Print and shaded views of the part. All mm, measured from the part's lowest x, y and z. Give positions to 0.01 mm unless a question says otherwise; leave off trailing zeros. Loops run counter-clockwise (first coordinate to the right, second up) from the corner with the lowest first, then second, coordinate; pieces in that order, holes last. Notation, with made-up numbers: (-7, -1.75) - (35, -1.75) arc R23 ccw to (35, 11.25) - close; hole circle Ø9 at (72, 4). An arc over 180 degrees is marked (long way). Return JSON: item names as keys, results as strings.
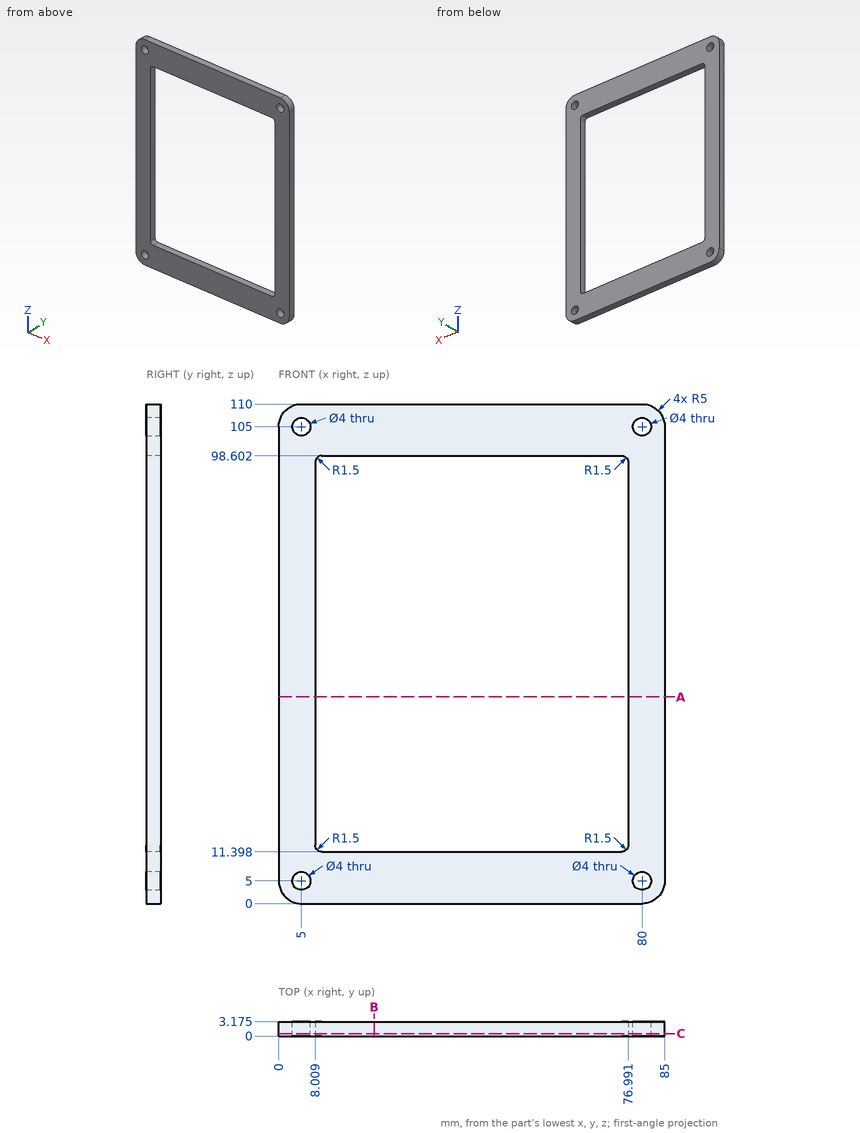
1. Cut at B-B, the plane x = 21. Write the cut outline in (y, z) (3 decimals).
Values follow:
{"outline": "(0, 0) - (3.175, 0) - (3.175, 11.398) - (0, 11.398) - close; (0, 98.602) - (3.175, 98.602) - (3.175, 110) - (0, 110) - close"}
2. Cut at A-A, the plane z = 45.5. Write the cut outline in (x, y) (3 decimals).
Values follow:
{"outline": "(0, 0) - (8.009, 0) - (8.009, 3.175) - (0, 3.175) - close; (76.991, 0) - (85, 0) - (85, 3.175) - (76.991, 3.175) - close"}
3. Cut at C-C, the plane y = 0.5. Write the cut outline in (x, z), plus the area to 3 significant figures.
Values follow:
{"outline": "(0, 5) arc R5 ccw to (5, 0) - (80, 0) arc R5 ccw to (85, 5) - (85, 105) arc R5 ccw to (80, 110) - (5, 110) arc R5 ccw to (0, 105) - close; hole circle Ø4 at (5, 5); hole circle Ø4 at (5, 105); hole (8.01, 12.9) arc R1.5 ccw to (9.51, 11.4) - (75.49, 11.4) arc R1.5 ccw to (76.99, 12.9) - (76.99, 97.1) arc R1.5 ccw to (75.49, 98.6) - (9.51, 98.6) arc R1.5 ccw to (8.01, 97.1) - close; hole circle Ø4 at (80, 5); hole circle Ø4 at (80, 105)", "area": "3,260 mm²"}
4. Drop a flat-ended pin along its axis: P1, Ø1.6, axis at x = 51, y = 2, coming from the -Z side. Give the stop position or say it passes through.
Values follow:
{"P1": "stops at z = 0"}
5. Drill centre lines: probe 1 along X at (y, z) = (1.55, 5); probe 2 along Z at (x, y) = (53.5, 2.6); probe 3 along X at (y, z) = (2.85, 42.5). Where is each one in solid material? Low to high.
Values follow:
{"probe 1": "x = 0 to 3, 7 to 78, 82 to 85", "probe 2": "z = 0 to 11.4, 98.6 to 110", "probe 3": "x = 0 to 8.01, 76.99 to 85"}
